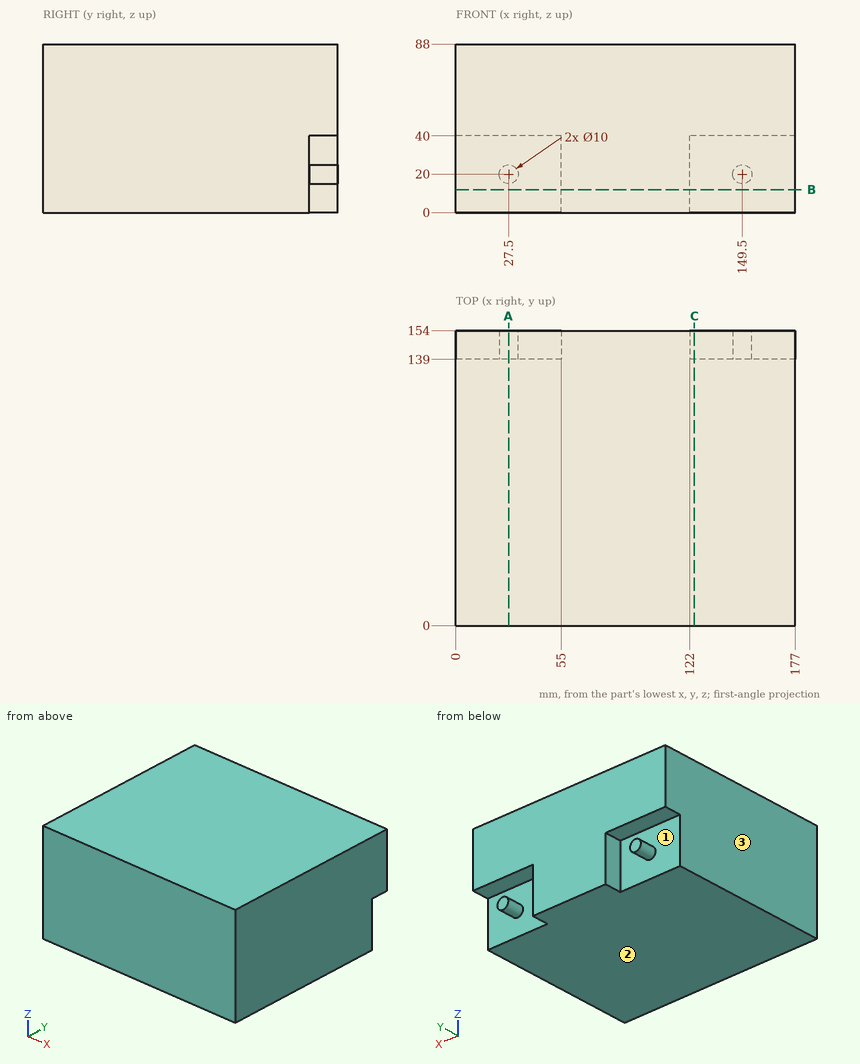
Here's the drawing with two shaded views (mm, measured from the low corner). I have some questions. Give positions to 0.01 mm unless a question says otherwise; leave off trailing zeros. Write each loop counter-clockwise with the first axis right and the second up, starting at its lowest first coordinate (ties: lowest second). Pieces come first, ordered by that corner, then holes. Notation, with made-up numbers: (60, -2) -> (102, -2) arc R21 cw to (102, 24) -> close; hole circle Ø10 at (-12.75, 78). An arc over 180 degrees is marked (long way). Use one line per item in the form item = value. Start each with the question number.
1. Thinking about a two-plate mould opening in X: for the marked faces 1, 2 and 3, which applies, +X half, -X half, draft (parallel to the pull), parting line (faces both ways), or undercut?
2. Will these pins go through, and if not, where does the flat tip stop? pin 1 Ø4.5 at (x, y) = (29, 150) entering from -Z; pin 2 Ø12 at (y, z) = (148.5, 27) entering from -X; pin 3 Ø4.5 at (y, z) = (148.5, 25.5) entering from +X.
3. Imagine slicing it at C-C on x = 124.5. List the corners of the cut face in (y, z) for me, plus the area to 3 significant figures.
4. Imagine slicing it at A-A on x = 27.5. List the corners of the cut face in (y, z) for me, plus the area to 3 significant figures.
5. If I drill on L1, parallel to Z at x = 150, y = 147; L2, parallel to Y at x = 158.5, z = 14, over which ranges is the centre line in solid material (lowest first)?
6. Imagine slicing it at B-B on z = 12. List the corners of the cut face in (x, y) for me.
Entries:
q1.face_1 = undercut
q1.face_2 = draft
q1.face_3 = -X half
q2.pin_1 = 15
q2.pin_2 = 22.6
q2.pin_3 = 153.3
q3.outline = (0, 0) -> (139, 0) -> (139, 40) -> (154, 40) -> (154, 88) -> (0, 88) -> close
q3.area = 13,000 mm²
q4.outline = (0, 0) -> (139, 0) -> (139, 15) -> (154, 15) -> (154, 25) -> (139, 25) -> (139, 40) -> (154, 40) -> (154, 88) -> (0, 88) -> close
q4.area = 13,100 mm²
q5.L1 = 15.03 to 24.97, 40 to 88
q5.L2 = 0 to 139
q6.outline = (0, 0) -> (177, 0) -> (177, 139) -> (122, 139) -> (122, 154) -> (55, 154) -> (55, 139) -> (0, 139) -> close
